Source: CAD feature listing. Evaluate the final solid. Frame: model axes, mm. Round coordinates to 2 decimals unless told otherwise and drop trailing zeros. Write each loop counter-clockwise with the first axis right and the second up, starting at its lowest first coordinate (ties: lowest second). Pieces come first, ordered by that corner, then holes. Notation, with made-up numbers: M 9.25,-34 L 15.25,-34 A9 ccw 15.25,-24 Z; hole C 74,-8 d5. An arc over 180 degrees is marked long. Answer in a Markdown table with one row per item.
from build123d import *

# Parameters (mm, degrees)
SKETCH1_R           = 2.5
BOSS_EXTRUDE1_DEPTH = 6


with BuildPart() as part:
    # Sketch1 → Boss-Extrude1 (new body)
    with BuildSketch(Plane.XY):
        with BuildLine():
            Line((0, -50), (158, -50))
            ThreePointArc((158, -50), (183, -25), (158, 0))
            Line((158, 0), (0, 0))
            Line((0, 0), (0, -50))
        make_face()
        with Locations((25, -25)):
            Circle(SKETCH1_R, mode=Mode.SUBTRACT)
        with Locations((158, -25)):
            Circle(SKETCH1_R, mode=Mode.SUBTRACT)
        with BuildLine():
            Line((50, -35), (130, -35))
            ThreePointArc((130, -35), (140, -25), (130, -15))
            Line((130, -15), (50, -15))
            ThreePointArc((50, -15), (40, -25), (50, -35))
        make_face(mode=Mode.SUBTRACT)
    extrude(amount=BOSS_EXTRUDE1_DEPTH)


solid = part.part
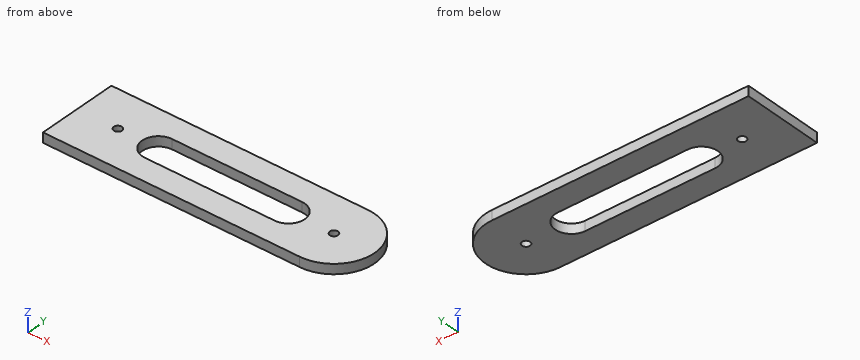
Q1. Material intervals for probe 1 along Y at (x, z) = (25, 3.8); probe 2 along Y at (x, z) = (95.5, 4.7); probe 3 along X at (y, z) = (-29, 2.75), sorted ascending.
Solutions:
| item | result |
|---|---|
| probe 1 | y = -50 to -27.5, -22.5 to 0 |
| probe 2 | y = -50 to -35, -15 to 0 |
| probe 3 | x = 0 to 40.83, 139.17 to 182.68 |
Q2. Section C-C (z = 4.6). Return loops of the section in (x, y), and give its area (3 significant figures).
Solutions:
| item | result |
|---|---|
| outline | M 0,-50 L 158,-50 A25 ccw 158,0 L 0,0 Z; hole C 25,-25 d5; hole M 50,-35 L 130,-35 A10 ccw 130,-15 L 50,-15 A10 ccw Z; hole C 158,-25 d5 |
| area | 6,930 mm2 |
Q3. Section B-B (y = -25). Return loops of the section in (x, z).
Solutions:
| item | result |
|---|---|
| outline | M 0,0 L 22.5,0 L 22.5,6 L 0,6 Z; M 27.5,0 L 40,0 L 40,6 L 27.5,6 Z; M 140,0 L 155.5,0 L 155.5,6 L 140,6 Z; M 160.5,0 L 183,0 L 183,6 L 160.5,6 Z |
Q4. Contact query for flat-ended pins moving along their axis: pin 1 Ø1.5 at (x, z) = (135.5, 4.5) entering from +Y; pin 2 Ø4 at (x, y) = (25, -25) entering from +Z. Output: stop coordinate, or through.
Solutions:
| item | result |
|---|---|
| pin 1 | stops at y = 0 |
| pin 2 | passes through |
Q5. Section D-D (x = 122). Return loops of the section in (y, z), and give its area (3 significant figures).
Solutions:
| item | result |
|---|---|
| outline | M -50,0 L -35,0 L -35,6 L -50,6 Z; M -15,0 L 0,0 L 0,6 L -15,6 Z |
| area | 180 mm2 |
Q6. Section A-A (x = 25). Return loops of the section in (y, z).
Solutions:
| item | result |
|---|---|
| outline | M -50,0 L -27.5,0 L -27.5,6 L -50,6 Z; M -22.5,0 L 0,0 L 0,6 L -22.5,6 Z |
